Can you work these out from the model? Positions are in its coordinate system, mm. A direction names the side the tool comes from. Give positions to 0.01 mm unless a question says otherwise; leave off trailing zeros. Order: outer loops, then holes, each group sorted by start corner. A loop starts at its lowest first (then second) coordinate and runs counter-clockwise, first axis right, second up. Notation, with made-up numbers: (27, 59) - (77, 59) arc R9 cw to (77, 72) - close; hole circle Ø10 at (83, 62). An arc over 180 degrees is marked (long way). Return JSON: item names as keys, results as strings.
```python
from build123d import *

# Parameters (mm, degrees)
F0_W     = 50
F0_H     = 50
F0_W_2   = 44
F0_H_2   = 44
F1_DEPTH = 1500
F2_DEPTH = 100
F3_R     = 5
F4_R     = 3
F6_DEPTH = 50


with BuildPart() as f1:
    # F0 (on Front) → F1 (new body)
    with BuildSketch(Plane.XZ):
        with Locations((25, 25)):
            Rectangle(F0_W, F0_H)
        with Locations((25, 25)):
            Rectangle(F0_W_2, F0_H_2, mode=Mode.SUBTRACT)
    extrude(amount=F1_DEPTH)

    # F0 (on Front) → F2 (join)
    with BuildSketch(Plane.XZ):
        with Locations((25, 25)):
            Rectangle(F0_W, F0_H)
        with Locations((25, 25)):
            Rectangle(F0_W_2, F0_H_2, mode=Mode.SUBTRACT)
    extrude(amount=F2_DEPTH)

    # F3
    f3_edges = [f1.edges().sort_by_distance(p)[0] for p in [
        (50, -750, 50),
        (50, -750, 0),
        (0, -750, 0),
        (0, -750, 50),
    ]]
    fillet(f3_edges, radius=F3_R)

    # F4
    f4_edges = [f1.edges().sort_by_distance(p)[0] for p in [
        (47, -750, 47),
        (3, -750, 3),
        (3, -750, 47),
        (47, -750, 3),
    ]]
    fillet(f4_edges, radius=F4_R)

    # F5 (on face) → F6 (cut)
    with BuildSketch(Plane.XY.offset(50)):
        Polygon((50, 0), (0, 0), (50, -50), align=None)
        Polygon((50, -1450), (0, -1500), (50, -1500), align=None)
    extrude(amount=-F6_DEPTH, mode=Mode.SUBTRACT)


solid = f1.part
```
1. Suppose I cut it at B-B (z = 16.5). List the corners of the cut face in (x, y) for me, plus the area to 3 significant figures.
Checks:
{"outline": "(0, -1500) - (3, -1497) - (3, -3) - (0, 0) - close; (47, -1453) - (50, -1450) - (50, -50) - (47, -47) - close", "area": "8,700 mm^2"}
2. If I drill on L1, parallel to Z at x = 15, y = -1344; L2, parallel to Z at x = 46, y = -446, over which ranges is the centre line in solid material (lowest first)? Write a range as [from, to].
Checks:
{"L1": "[0, 3], [47, 50]", "L2": "[0.1, 3.76], [46.24, 49.9]"}
3. On a 3-axis mill with a long thin cutter (end or side, diameter ignored), from which of +Z, -Z, +X, -X, +Y, -Y can I reach the whole of each face in a straight line? I mean faces 1 (the face through (50, -740, 25)), 2 (the face through (47, -740, 25)). Say none if no direction works.
Checks:
{"face 1": "+Z, -Z, +X, +Y, -Y", "face 2": "+Y, -Y"}
4. Suppose I cut it at A-A (x = 22). List the corners of the cut face in (y, z) for me, plus the area to 3 significant figures.
Checks:
{"outline": "(-1478, 0) - (-22, 0) - (-22, 3) - (-1478, 3) - close; (-1478, 47) - (-22, 47) - (-22, 50) - (-1478, 50) - close", "area": "8,740 mm^2"}
5. Suppose I cut it at C-C (y = -800). List the corners of the cut face in (x, z) for me, plus the area to 3 significant figures.
Checks:
{"outline": "(0, 5) arc R5 ccw to (5, 0) - (45, 0) arc R5 ccw to (50, 5) - (50, 45) arc R5 ccw to (45, 50) - (5, 50) arc R5 ccw to (0, 45) - close; hole (3, 6) arc R3 ccw to (6, 3) - (44, 3) arc R3 ccw to (47, 6) - (47, 44) arc R3 ccw to (44, 47) - (6, 47) arc R3 ccw to (3, 44) - close", "area": "550 mm^2"}
6. Thinking about a two-plate mould opening in Z: for faces 3 (the face through (25.1, -1474.9, 47.3)), 4 (the face through (25, -740, 0)), 5 (the face through (25, -740, 50)), 6 (the face through (3, -740, 25)), which applies, +Z half, -Z half, draft (parallel to the pull), parting line (faces both ways), or undercut?
Checks:
{"face 3": "draft", "face 4": "-Z half", "face 5": "+Z half", "face 6": "undercut"}
